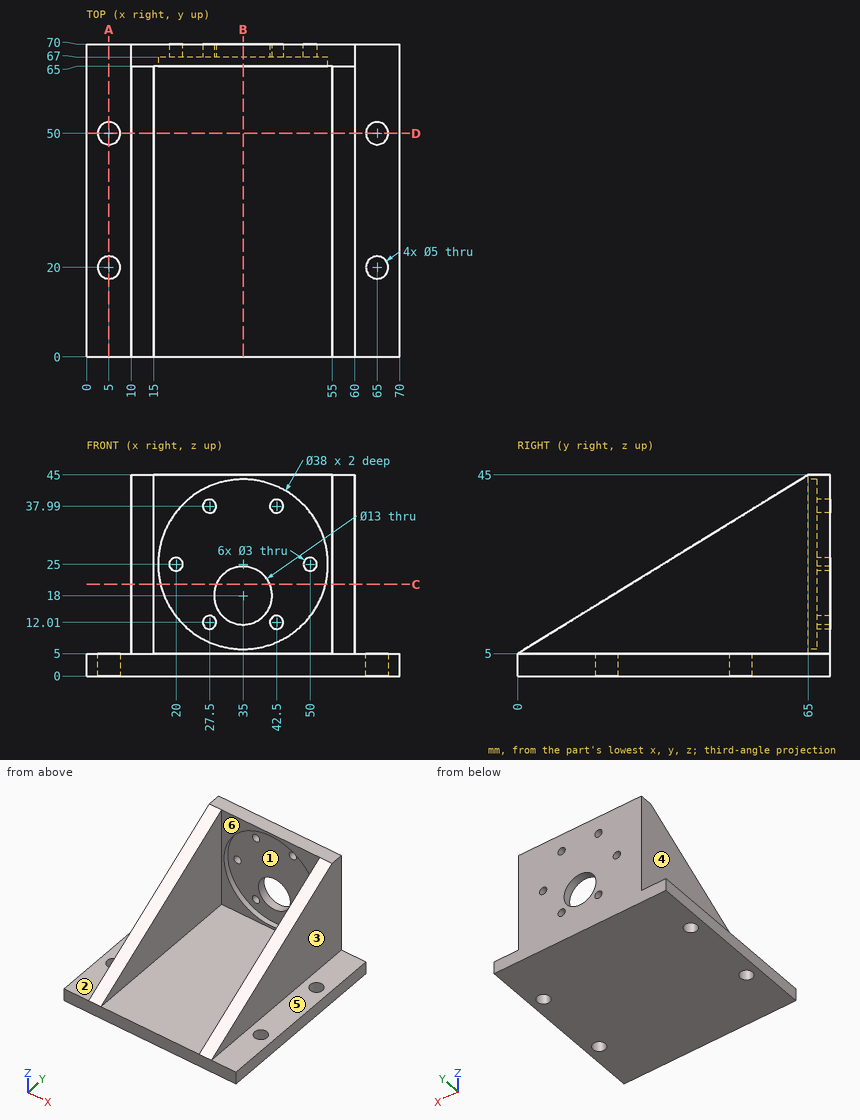
Geometry check sheet. Reference: drawing and pictorial views, mm from the part's lowest x, y, z. A direction names the side the tool comes from. Give positions to 0.01 mm unless a question says otherwise; leave off trailing zeros. Write each loop counter-clockwise with the first axis right and the second up, starting at its lowest first coordinate (ties: lowest second). Pieces come first, ordered by that corner, then holes. Notation, with made-up numbers: M 34,81.25 L 90,81.25 A8 ccw 90,94.25 Z; hole C 71.25,19.25 d2. An arc over 180 degrees is marked long. Answer as CSV lines item,"result". Start each with the question number.
Q1. Material ranges on L1, parallel to X at y = 62.5, z = 24.5; L2, parallel to Z at x = 42.5, y = 67.75; L3, parallel to Y at x = 65, z = 1.95, recorded low to high.
Q2. Section check D-D, the plane y = 50. Record the cut outline in (x, z).
Q3. Section check A-A, the plane x = 5. Record the cut outline in (y, z), then the cut area to 3 significant figures.
Q4. Tool access check on the marked faces 4, 5 and 6. Record the directions out of +Z, -Z, +X, -X, +Y, -Y that give a thin tool (end or side, any length) a straight path to the whole face; none if there is none.
Q5. Go/stop test with flat-tipped pins: pin 1 (5 mm diameter, centred on x = 63.5, y = 44.5, fed in from +Z); pin 2 (5 mm diameter, centred on x = 22.5, z = 30.5, fed in from -Y); pin 3 (20 mm diameter, centred on y = 40.5, z = 20.5, fed in from -X); pin 4 (1 mm diameter, centred on x = 7.5, y = 26, fed in from -Z). Record where each tip stops, or that it passes through.
Q6. Release check for a two-part mould opening along X. For the marked faces 1, 2 and 3 record: pulls with the +X half, pulls with the -X half, needs draft (parallel to the pull), parting line crosses it, or undercut.
Q7. Section check B-B, the plane x = 35. Record the cut outline in (y, z), then the cut area to 3 significant figures.
Q8. Section check C-C, the plane z = 20.5. Record the cut outline in (x, y).
Geometry says:
1,L1,"10 to 15, 55 to 60"
1,L2,"0 to 10.51, 13.51 to 36.49, 39.49 to 45"
1,L3,"0 to 17.5, 22.5 to 47.5, 52.5 to 70"
2,outline,"M 0,0 L 2.5,0 L 2.5,5 L 0,5 Z; M 7.5,0 L 62.5,0 L 62.5,5 L 60,5 L 60,35.77 L 55,35.77 L 55,5 L 15,5 L 15,35.77 L 10,35.77 L 10,5 L 7.5,5 Z; M 67.5,0 L 70,0 L 70,5 L 67.5,5 Z"
3,outline,"M 0,0 L 17.5,0 L 17.5,5 L 0,5 Z; M 22.5,0 L 47.5,0 L 47.5,5 L 22.5,5 Z; M 52.5,0 L 70,0 L 70,5 L 52.5,5 Z"
3,area,"300 mm^2"
4,face 4,"+Z, -X, +Y, -Y"
4,face 5,"+Z, +X, +Y, -Y"
4,face 6,"+Z, -Y"
5,pin 1,"z = 5"
5,pin 2,"y = 67"
5,pin 3,"x = 10"
5,pin 4,"z = 0"
6,face 1,"undercut"
6,face 2,"needs draft"
6,face 3,"pulls with the +X half"
7,outline,"M 0,0 L 70,0 L 70,11.5 L 67,11.5 L 67,6 L 65,6 L 65,5 L 0,5 Z; M 65,44 L 67,44 L 67,24.5 L 70,24.5 L 70,45 L 65,45 Z"
7,area,"435 mm^2"
8,outline,"M 10,25.19 L 15,25.19 L 15,65 L 16.54,65 L 16.54,67 L 29,67 L 29,70 L 10,70 Z; M 41,67 L 53.46,67 L 53.46,65 L 55,65 L 55,25.19 L 60,25.19 L 60,70 L 41,70 Z"
